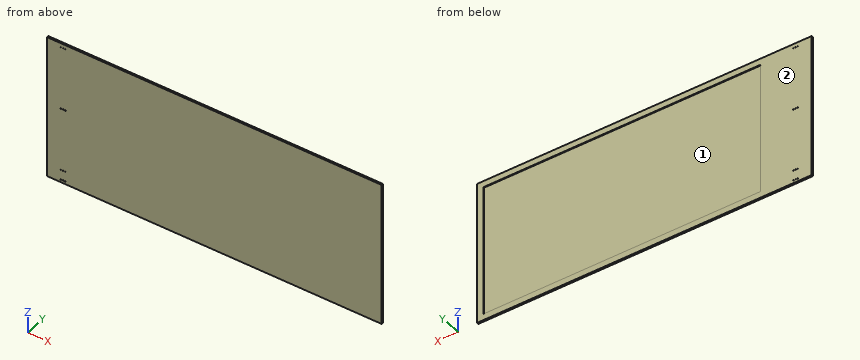
from build123d import *

# Parameters (mm, degrees)
SKETCH1_W           = 1066.8
SKETCH1_H           = 508
BOSS_EXTRUDE1_DEPTH = 6.35
SKETCH2_W           = 919.1625
SKETCH2_H           = 463.55
CUT_EXTRUDE1_DEPTH  = 3.175
SKETCH3_R           = 1.3589
CUT_EXTRUDE2_DEPTH  = 7.35
SKETCH5_W           = 55.9181
SKETCH5_H           = 463.55
BOSS_EXTRUDE2_DEPTH = 2.54
SKETCH6_W           = 116.2812
SKETCH6_H           = 508
BOSS_EXTRUDE3_DEPTH = 6.35
SKETCH7_W           = 116.2812
SKETCH7_H           = 463.55
CUT_EXTRUDE3_DEPTH  = 3.175


with BuildPart() as part:
    # Sketch1 → Boss-Extrude1 (new body)
    with BuildSketch(Plane(origin=(0, 0, 0), x_dir=(1, 0, 0), z_dir=(0, 1, 0))):
        with Locations((533.4, 254)):
            Rectangle(SKETCH1_W, SKETCH1_H)
    extrude(amount=BOSS_EXTRUDE1_DEPTH)

    # Sketch2 → Cut-Extrude1 (cut)
    with BuildSketch(Plane(origin=(0, 6.35, 0), x_dir=(1, 0, 0), z_dir=(0, 1, 0))):
        with Locations((584.99375, 254)):
            Rectangle(SKETCH2_W, SKETCH2_H)
    extrude(amount=-CUT_EXTRUDE1_DEPTH, mode=Mode.SUBTRACT)

    # Sketch3 → Cut-Extrude2 (cut, through all)
    with BuildSketch(Plane(origin=(0, 6.35, 0), x_dir=(1, 0, 0), z_dir=(0, 1, 0))):
        with Locations((49.149, 462.4832)):
            Circle(SKETCH3_R)
        with Locations((49.149, 498.094)):
            Circle(SKETCH3_R)
        with Locations((56.8452, 498.094)):
            Circle(SKETCH3_R)
        with Locations((56.8452, 462.4832)):
            Circle(SKETCH3_R)
        with Locations((64.5414, 498.094)):
            Circle(SKETCH3_R)
        with Locations((64.5414, 462.4832)):
            Circle(SKETCH3_R)
        with Locations((49.149, 14.8082)):
            Circle(SKETCH3_R)
        with Locations((57.0992, 14.8082)):
            Circle(SKETCH3_R)
        with Locations((65.0494, 14.8082)):
            Circle(SKETCH3_R)
        with Locations((49.149, 238.6457)):
            Circle(SKETCH3_R)
        with Locations((57.0992, 238.6457)):
            Circle(SKETCH3_R)
        with Locations((65.0494, 238.6457)):
            Circle(SKETCH3_R)
    extrude(amount=-CUT_EXTRUDE2_DEPTH, mode=Mode.SUBTRACT)

    # Sketch5 → Boss-Extrude2 (add)
    with BuildSketch(Plane(origin=(0, 6.35, 0), x_dir=(1, 0, 0), z_dir=(0, 1, 0))):
        with Locations((153.37155, 254)):
            Rectangle(SKETCH5_W, SKETCH5_H)
    extrude(amount=-BOSS_EXTRUDE2_DEPTH)

    # Sketch6 → Boss-Extrude3 (add)
    with BuildSketch(Plane(origin=(0, 6.35, 0), x_dir=(1, 0, 0), z_dir=(0, 1, 0))):
        with Locations((1124.9406, 254)):
            Rectangle(SKETCH6_W, SKETCH6_H)
    extrude(amount=-BOSS_EXTRUDE3_DEPTH)

    # Sketch7 → Cut-Extrude3 (cut)
    with BuildSketch(Plane(origin=(0, 6.35, 0), x_dir=(1, 0, 0), z_dir=(0, 1, 0))):
        with Locations((1102.7156, 254)):
            Rectangle(SKETCH7_W, SKETCH7_H)
    extrude(amount=-CUT_EXTRUDE3_DEPTH, mode=Mode.SUBTRACT)


solid = part.part
Here's how the part is built. I have some questions about the finished solid (model axes, mm). Face numbers are marked on the shaded views. Coordinates: 2 decimals unless noted, no trailing zeros. Order: outer loops, then holes, each group sorted by start corner. A loop starts at its lowest first (then second) coordinate and runs counter-clockwise, first axis right, second up. Notation, with made-up numbers: (-31, 47) -> (22, 47) arc R19 ccw to (22, 67) -> close; hole circle Ø1 at (20.25, -24.75). An arc over 180 degrees is marked (long way). Answer in a Markdown table with one row per item.
(1) I want a section at A-A on x = 1083. List the corners of the cut face in (y, z) for me (3 decimals), then the cut area to 3 significant figures.
Answer key:
| item | result |
|---|---|
| outline | (0, -508) -> (6.35, -508) -> (6.35, -485.775) -> (3.175, -485.775) -> (3.175, -22.225) -> (6.35, -22.225) -> (6.35, 0) -> (0, 0) -> close |
| area | 1,750 mm^2 |
(2) Thinking about a two-plate mould opening in Z: for the marked faces 1 and 2, which applies, +Z half, -Z half, draft (parallel to the pull), parting line (faces both ways), or undercut?
Answer key:
| item | result |
|---|---|
| face 1 | undercut |
| face 2 | draft |
(3) Please list where these lines run through material, in increasing order: probe 1 along Y at (x, z) = (164.5, -316) (3 decimals); probe 2 along X at (y, z) = (5.25, -405.5); probe 3 along Z at (x, y) = (214.5, 4.75) (3 decimals).
Answer key:
| item | result |
|---|---|
| probe 1 | 0 to 3.175, 3.81 to 6.35 |
| probe 2 | 0 to 181.33, 1160.86 to 1183.08 |
| probe 3 | -508 to -485.775, -22.225 to 0 |
(4) Will this pin go through, and if not, where does the flat tip stop? pin 1 Ø1.5 at (x, z) = (897.5, -280.5) entering from +Y (3 decimals).
Answer key:
| item | result |
|---|---|
| pin 1 | y = 3.175 |
